Autodesk Inventor part; units mm, degrees
ref_plane "Płaszczyzna konstrukcyjna1" through (102.5, 425.9063, 229.6758) normal (0, 0, -1) x (-1, 0, 0)
ref_plane "Płaszczyzna konstrukcyjna2" through (102.5, 425.9063, 41.6758) normal (0, -1, 0) x (1, 0, 0)
ref_plane "YZ Plane" through (0, 0, 0) normal (1, 0, 0) x (0, 1, 0)
sketch "Szkic1" plane through (0, 0, 0) normal (1, 0, 0) x (0, 1, 0)
  circle A0 centre (425.9063, 179.6758) radius 4.1
  line L0 (460.0949, 39.6758) -> (391.7177, 39.6758)
  line L1 (428.4063, 86.5216) -> (428.4063, 97.3591)
  line L2 (428.4063, 97.3591) -> (423.4063, 97.3591)
  line L3 (423.4063, 97.3591) -> (423.4063, 86.5216)
  arc A1 (423.4063, 86.5216) -> (428.4063, 86.5216) centre (425.9063, 77.8758) ccw
  circle A2 centre (406.1366, 78.0058) radius 1.65
  line L4 (460.0949, 143.191) -> (460.0949, 39.6758)
  arc A3 (460.0949, 143.191) -> (391.7177, 143.191) centre (425.9063, 179.6758) ccw
  line L5 (391.7177, 39.6758) -> (391.7177, 143.191)
  circle A4 centre (449.4563, 101.4258) radius 2.6
  circle A5 centre (402.3563, 101.4258) radius 2.6
  circle A6 centre (402.3563, 54.3258) radius 2.6
  circle A7 centre (449.4563, 54.3258) radius 2.6
  line L6 (423.4063, 95.8758) -> (428.4063, 95.8758)
  point P0 (0, 0)
  point P1 (391.7177, 143.191)
  dimension "d0" = 5.2
  dimension "d1" = 50
  dimension "d2" = 8.2
  dimension "d3" = 9
  dimension "d4" = 3.3
  dimension "d5" = 31.6886
  dimension "d6" = 36.6886
  dimension "d7" = 68.3772
  dimension "d8" = 1.4833
  dimension "d9" = 57.6833
  dimension "d10" = 0
  dimension "d11" = 45.8319
  dimension "d12" = 45.8319
  dimension "d13" = 57.6833
  dimension "d14" = 0
  dimension "d15" = 10.6386
  dimension "d16" = 4.0667
  dimension "d17" = 10.6386
  dimension "d18" = 43.0333
  dimension "d19" = 31.6886
  dimension "d20" = 0
  dimension "d21" = 31.6886
  dimension "d22" = 10.8375
  dimension "d23" = 31.6886
  dimension "d24" = 10.8375
  dimension "d25" = 34.1886
  dimension "d26" = 34.1886
  dimension "d27" = 36.6886
  dimension "d28" = 0
  dimension "d29" = 36.6886
  dimension "d30" = 10.8375
  dimension "d31" = 36.6886
  dimension "d32" = 22.2697
  dimension "d33" = 19.3533
  dimension "d34" = 57.7386
  dimension "d35" = 4.0667
  dimension "d36" = 57.7386
  dimension "d37" = 43.0333
  dimension "d38" = 68.3772
  dimension "d39" = 45.8319
  dimension "d40" = 68.3772
  dimension "d41" = 57.6833
extrude "Wyciągnięcie proste1" add sketch "Szkic1" along normal blind 102.5
ref_plane "Płaszczyzna konstrukcyjna1" through (102.5, 425.9063, 229.6758) normal (0, 0, -1) x (-1, 0, 0)
sketch "Szkic2" plane through (102.5, 425.9063, 229.6758) normal (0, 0, -1) x (-1, 0, 0)
  line L0 (102.5, 50) -> (0, 50)
  line L1 (99.5, 50) -> (99.5, -50)
  line L2 (102.5, -50) -> (0, -50)
  line L3 (3, 50) -> (3, -50)
  line L4 (102.5, 50) -> (102.5, -50)
  line L5 (0, 50) -> (0, -50)
  line L6 (99.5, 50) -> (3, 50)
  line L7 (3, -50) -> (99.5, -50)
  point P0 (102.5, -425.9063)
  point P1 (102.5, 34.1886)
  point P2 (102.5, -34.1886)
  point P3 (0, 34.1886)
  point P4 (0, -34.1886)
  point P5 (3, 50)
  dimension "d44" = 3
  dimension "d45" = 3
extrude "Wyciągnięcie proste2" cut sketch "Szkic2" along normal blind 187 contours L1 L2 L3 L0
fillet "Zaokrąglenie1" radius 2 2 edges at (0, 425.9063, 39.6758) (102.5, 425.9063, 39.6758)
sketch "Szkic3" plane through (102.5, 0, 0) normal (1, 0, 0) x (0, 0, -1)
  circle A0 centre (-179.6758, 425.9063) radius 4.1
  circle A1 centre (-179.6758, 425.9063) radius 50
  line L0 (-143.0152, 391.9063) -> (-39.6758, 391.9063)
  line L1 (-39.6758, 391.7177) -> (-39.6758, 460.0949)
  line L2 (-143.0152, 459.9063) -> (-39.6758, 459.9063)
  line L3 (-39.6758, 425.9063) -> (-57.2336, 425.9063)
  line L4 (-143.191, 391.7177) -> (-41.6758, 391.7177)
  line L5 (-41.6758, 460.0949) -> (-143.191, 460.0949)
  line L6 (-39.6758, 391.7177) -> (-41.6758, 391.7177)
  line L7 (-41.6758, 460.0949) -> (-39.6758, 460.0949)
  point P0 (0, 0)
  dimension "d49" = 68
  dimension "d50" = 34
  dimension "d51" = 100
extrude "Wyciągnięcie proste3" cut sketch "Szkic3" against normal through all contours A1 L5 L7 L1 L2 | L0 L1 L6 L4 A1
sketch "Szkic4" plane through (102.5, 459.9063, 143.0152) normal (0, 1, 0) x (1, 0, 0)
  line L0 (-3, 100.3394) -> (-99.5, 100.3394)
  line L1 (-100.5, 103.3394) -> (-2, 103.3394)
  line L2 (-3, 100.3394) -> (-3, 103.3394)
  line L3 (-2, 103.3394) -> (-100.5, 103.3394)
  line L4 (0, 101.3394) -> (0, 0)
  line L5 (-99.5, 100.3394) -> (-99.5, 103.3394)
  point P0 (-102.5, 143.0152)
  point P1 (-3, 103.3394)
  dimension "d54" = 3
extrude "Wyciągnięcie proste4" add sketch "Szkic4" along normal blind 3
ref_plane "Płaszczyzna konstrukcyjna2" through (102.5, 425.9063, 41.6758) normal (0, -1, 0) x (1, 0, 0)
mirror "Odbij1" about plane through (102.5, 425.9063, 41.6758) normal (0, -1, 0) of "Wyciągnięcie proste4"
sketch "Szkic5" plane through (2, 391.9063, 39.6758) normal (0, 0, -1) x (-1, 0, 0)
  line L0 (-1, 71) -> (-97.5, 71)
  line L1 (-97.5, 71) -> (-97.5, 74)
  line L2 (-97.5, -16) -> (-97.5, 84)
  line L3 (-97.5, 74) -> (-1, 74)
  line L4 (-1, -16) -> (-1, 84)
  line L5 (-1, 74) -> (-1, 71)
  line L6 (-1, 71) -> (-97.5, 71)
  line L7 (-97.5, 0) -> (-1, 0)
  line L8 (-1, 0) -> (-1, -3)
  line L9 (-1, -3) -> (-97.5, -3)
  line L10 (-97.5, -3) -> (-97.5, 0)
  point P0 (2, -391.9063)
  point P1 (-97.5, 68)
  point P2 (-1, 68)
  dimension "d57" = 3
  dimension "d58" = 3
extrude "Wyciągnięcie proste5" add sketch "Szkic5" against normal blind 71 contours L0 L1 L3 L4
mirror "Odbij2" about plane through (102.5, 425.9063, 41.6758) normal (0, -1, 0) of "Wyciągnięcie proste5"
fillet "Zaokrąglenie2" radius 2 2 edges at (51.25, 465.9063, 39.6758) (51.25, 385.9063, 39.6758)
sketch "Szkic6" plane through (3, 385.9063, 110.6758) normal (0, -1, 0) x (1, 0, 0)
  circle A0 centre (85.5, -6) radius 2.85
  circle A1 centre (11, -6) radius 2.85
  line L0 (0, -69) -> (0, 0)
  line L1 (0, -71) -> (96.5, -71)
  line L2 (96.5, -69) -> (96.5, 0)
  point P0 (-3, -110.6758)
  dimension "d62" = 5.7
  dimension "d63" = 5.7
  dimension "d64" = 11
  dimension "d65" = 65
  dimension "d66" = 11
  dimension "d67" = 65
extrude "Wyciągnięcie proste6" cut sketch "Szkic6" against normal through all
sketch "Szkic7" plane through (99.5, 425.9063, 179.6758) normal (-1, 0, 0) x (0, 0, 1)
  circle A0 centre (-78.25, -23.55) radius 2.6
  circle A1 centre (-78.25, -23.55) radius 6
  point P0 (-179.6758, -425.9063)
  dimension "d70" = 12
chamfer "Faza1" distance 2 angle 45 1 edges at (99.5, 399.7563, 101.4258)
chamfer "Faza2" distance 2 angle 45 1 edges at (3, 399.7563, 101.4258)
sketch "Szkic8" plane through (102.5, 0, 0) normal (1, 0, 0) x (0, 0, -1)
  point P0 (-190.9258, 406.4207)
  point P1 (-190.9258, 445.3919)
  point P2 (-157.1758, 425.9063)
hole "Otwór1" at (102.5, 406.4207, 190.9258) at (102.5, 445.3919, 190.9258) at (102.5, 425.9063, 157.1758) direction (-1, 0, 0) diameter 2.459 depth 4.25 tip angle 120
sketch "Szkic9" plane through (2, 391.9063, 39.6758) normal (0, 0, -1) x (-1, 0, 0)
  circle A0 centre (-49.25, 34) radius 4
  line L0 (-1, 74) -> (-97.5, 74)
  line L1 (-100.5, 68) -> (-100.5, 0)
  line L2 (-49.25, 34) -> (-93.3771, 34)
  line L3 (-49.25, 34) -> (-49.25, 64.9059)
  circle A1 centre (-87.25, 34) radius 3
  circle A2 centre (-49.25, 59) radius 3
  circle A3 centre (-11.25, 34) radius 3
  circle A4 centre (-49.25, 9) radius 3
  point P0 (2, -391.9063)
  dimension "d84" = 8
  dimension "d85" = 40
  dimension "d86" = 51.25
  dimension "d89" = 6
  dimension "d90" = 6
  dimension "d91" = 38
  dimension "d92" = 25
  dimension "d93" = 6
  dimension "d94" = 38
  dimension "d95" = 6
  dimension "d96" = 25
extrude "Wyciągnięcie proste7" cut sketch "Szkic9" against normal blind 71
sketch "Szkic10" plane through (0, 0, 0) normal (-1, 0, 0) x (0, 0, 1)
  point P0 (190.9258, 406.4207)
  point P1 (157.1758, 425.9063)
  point P2 (190.9258, 445.3919)
hole "Otwór2" at (0, 406.4207, 190.9258) at (0, 425.9063, 157.1758) at (0, 445.3919, 190.9258) direction (1, 0, 0) diameter 2.459 depth 4.25 tip angle 120
sketch "Szkic11" plane through (102.5, 0, 0) normal (1, 0, 0) x (0, 0, -1)
  circle A0 centre (-190.9258, 445.3919) radius 1.2295
  circle A1 centre (-190.9258, 445.3919) radius 1.2295
  circle A2 centre (-179.6758, 425.9063) radius 4.1
  circle A3 centre (-179.6758, 425.9063) radius 4.1
  point P0 (0, 0)
equation "\"PromieńGięcia\" = Grubość"
equation "\"SzerokośćGięciaPodcięcia\" = Grubość"
equation "\"GłębokośćGięciaPodcięcia\" = 0.5 * Grubość"
equation "\"RozmiarPodcięciaNarożnika\" = 4 * Grubość"
equation "\"MinimalnaPozostałość\" = 2 * Grubość"
equation "\"PromieńPrzejścia\" = PromieńGięcia"
equation "\"Rozmiar_promienia_Jacobiego\" = PromieńGięcia"
equation "\"Wielk_odstępu\" = Grubość"
properties part number "wzmocnienie2M1Dedit"
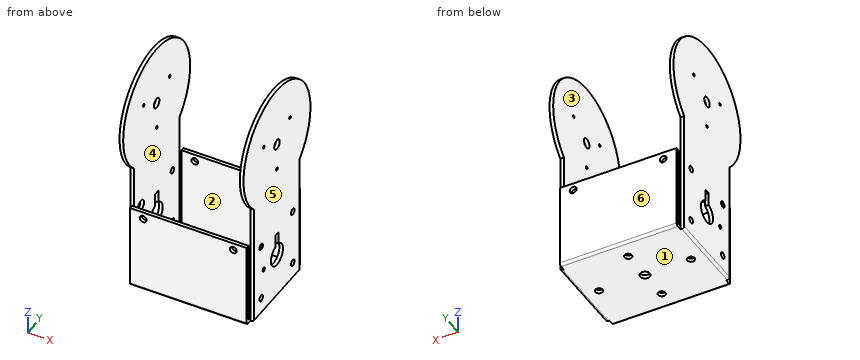
Design review of the part built by this model. Coordinates are the model's own, in mm. Face numbers are marked on the shaded views. A direction names the side the tool comes from. Give positions to 0.01 mm unless a question says otherwise; leave off trailing zeros. Order: outer loops, then holes, each group sorted by start corner. A loop starts at its lowest first (then second) coordinate and runs counter-clockwise, first axis right, second up. Notation, with made-up numbers: (29, 77.25) - (36, 77.25) arc R28 ccw to (36, 113.25) - close; hole circle Ø7 at (-18.75, -27.75). An arc over 180 degrees is marked (long way). Use a Markdown table: item, result. Add a question column.
(1) Add section D-D on z = 94.5. Give the boundary of the cut face in (x, y).
(2) Add section C-C on y = 419.5. Give the boundary of the cut face in (x, z), then the cut area to 3 significant figures.
(3) Mouldability with a two-part tool opening along Y and no side actions: class the marked faces 4, 5 and 6 as +Y half, -Y half, draft (parallel to the pull), parting line (faces both ways), or undercut.
(4) Wall thickness on probe 1 along X at (y, z) = (412, 75.5); probe 2 along Z at (x, y) = (48.5, 448); probe 3 along Y at (x, z) = (55.5, 102): over which ranges is each line inside the solid? List them lowest first. Write a range as [from, to].
(5) Add section B-B on x = 88.5. Give the boundary of the cut face in (y, z), then the cut area to 3 significant figures.
(6) Clearance check with flat-ended pins moving along their axes: P1, Ø2.5, axis at x = 1.5, z = 89.5, coming from the +Y side; P2, Ø4, axis at x = 49, y = 386, coming from the +Z side; P3, Ø3.5, axis at x = 101.5, z = 91.5, coming from the -Y side. State where each tip first meets the part, or that it passes through.
(7) Add section A-A on z = 64.5. Give the boundary of the cut face in (x, y).
(8) Machinability: for the marked faces 1, 2 and 3, which of the approach directions +Z, -Z, +X, -X, +Y, -Y give a long, thin tool a straight path to every point of the face, cutting with its end or side? Answer none if there is none.
Report:
| question | item | result |
|---|---|---|
| 1 | outline | (0, 391.91) - (3, 391.91) - (3, 423.41) - (0, 423.41) - close; (0, 428.41) - (3, 428.41) - (3, 459.91) - (0, 459.91) - close; (3, 385.91) - (99.5, 385.91) - (99.5, 388.91) - (3, 388.91) - close; (3, 462.91) - (99.5, 462.91) - (99.5, 465.91) - (3, 465.91) - close; (99.5, 391.91) - (102.5, 391.91) - (102.5, 423.41) - (99.5, 423.41) - close; (99.5, 428.41) - (102.5, 428.41) - (102.5, 459.91) - (99.5, 459.91) - close |
| 2 | outline | (0, 41.68) arc R2 ccw to (2, 39.68) - (100.5, 39.68) arc R2 ccw to (102.5, 41.68) - (102.5, 71.55) - (99.5, 71.55) - (99.5, 42.68) - (3, 42.68) - (3, 71.55) - (0, 71.55) - close; (0, 84.2) - (3, 84.2) - (3, 229.26) - (0, 229.26) - close; (99.5, 84.2) - (102.5, 84.2) - (102.5, 229.26) - (99.5, 229.26) - close |
| 2 | area | 1,350 mm² |
| 3 | face 4 | undercut |
| 3 | face 5 | draft |
| 3 | face 6 | +Y half |
| 4 | probe 1 | x = [0, 3], [99.5, 102.5] |
| 4 | probe 2 | z = [39.68, 42.68] |
| 4 | probe 3 | y = [385.91, 388.91], [462.91, 465.91] |
| 5 | outline | (385.91, 41.68) arc R2 ccw to (387.91, 39.68) - (423, 39.68) - (423, 42.68) - (388.91, 42.68) - (388.91, 101.83) - (385.91, 101.83) - close; (385.91, 107.53) - (388.91, 107.53) - (388.91, 110.68) - (385.91, 110.68) - close; (428.81, 39.68) - (463.91, 39.68) arc R2 ccw to (465.91, 41.68) - (465.91, 101.83) - (462.91, 101.83) - (462.91, 42.68) - (428.81, 42.68) - close; (462.91, 107.53) - (465.91, 107.53) - (465.91, 110.68) - (462.91, 110.68) - close |
| 5 | area | 595 mm² |
| 6 | P1 | stops at y = 459.91 |
| 6 | P2 | stops at z = 110.68 |
| 6 | P3 | stops at y = 391.91 |
| 7 | outline | (0, 391.91) - (3, 391.91) - (3, 459.91) - (0, 459.91) - close; (3, 385.91) - (99.5, 385.91) - (99.5, 388.91) - (3, 388.91) - close; (3, 462.91) - (99.5, 462.91) - (99.5, 465.91) - (3, 465.91) - close; (99.5, 391.91) - (102.5, 391.91) - (102.5, 459.91) - (99.5, 459.91) - close |
| 8 | face 1 | -Z, +X, -X, +Y, -Y |
| 8 | face 2 | +Z, +X, -X |
| 8 | face 3 | +Z |
